Autodesk Inventor part; units mm, degrees
ref_plane "YZ Plane" through (0, 0, 0) normal (1, 0, 0) x (0, 1, 0)
ref_plane "XZ Plane" through (0, 0, 0) normal (0, 1, 0) x (-1, 0, 0)
ref_plane "XY Plane" through (0, 0, 0) normal (0, 0, 1) x (1, 0, 0)
sketch "Esquisse2" plane through (0, 0, 0) normal (1, 0, 0) x (0, 1, 0)
  line L0 (0, 0) -> (0, -2.1683)
  line L1 (0, 0) -> (0, 50)
  line L2 (0, 0) -> (1.5, 0)
  line L3 (1.5, 0) -> (1.5, 5)
  line L4 (1.5, 5) -> (2.5, 5)
  line L5 (2.5, 5) -> (2.5, 10)
  line L6 (2.5, 10) -> (1.5, 10)
  line L7 (1.5, 10) -> (1.5, 50)
  line L8 (0, 50) -> (1.5, 50)
  dimension "d0" = 3
  dimension "d1" = 1
  dimension "d2" = 5
  dimension "d3" = 5
  dimension "d4" = 40
revolve "Révolution1" add sketch "Esquisse2" angle 360 about axis through (0, 0, 0) along (0, 0, -1)
thread "Filetage1"
chamfer "Chanfrein1" distance 0.5 angle 45 1 edges at (0, -1.5, 0)
properties part number "piston_axe"
The model under review builds one solid part; all positions refer to its coordinate system, in mm. A direction names the side the tool comes from. Coordinates: 2 decimals unless noted, no trailing zeros. Write each loop counter-clockwise with the first axis right and the second up, starting at its lowest first coordinate (ties: lowest second). Pieces come first, ordered by that corner, then holes. Notation, with made-up numbers: (75, 78) -> (113, 78) arc R15 ccw to (113, 82) -> close; hole circle Ø7 at (69.25, 66). An arc over 180 degrees is marked (long way). One line per item, written item: value. Start each with the question number.
Q1. To check wall thickness, follow probe 1 along Y at (x, z) = (0.05, 46.5); probe 2 along Z at (x, y) = (-1.5, 1.35); probe 3 along X at (y, z) = (-0.55, 25). State the ranges of each line that lie inside material, in increasing order.
Q2. For faces 3 (the face through (0, 2, 5)), 4 (the face through (0, 0, 50)), 5 (the face through (0, 2, 10)), list the 3-axis set-ups (+Z, -Z, +X, -X, +Y, -Y) from which the entire face can be reached by the end or side of a thin tool; tool diameter is ignored.
Q3. Add section A-A, the plane y = 0. Give the boundary of the cut face in (x, z).
Q4. The part is to be moulded in two halves that separate along Y. For faces 1 (the face through (0, 0, 0)), 2 (the face through (2.44, -0.54, 7.54)), say which applies: +Y half, -Y half, draft (parallel to the pull), parting line (faces both ways), or undercut.
Q5. Add section C-C, the plane z = 27. Give the boundary of the cut face in (x, y).
Q6. Add section D-D, the plane x = -2. Give the boundary of the cut face in (y, z), then the cut area to 3 significant figures.
Q7. Clearance check with flat-ended pins moving along their axes: P1, Ø2, axis at x = 2, z = 16.5, coming from the -Y side; P2, Ø3, axis at y = 0.5, z = 39.5, coming from the -X side; P3, Ø1.5, axis at x = 1, z = 29, coming from the -Y side. State where each tip first meets the part, or that it passes through.
Response:
1. probe 1: -1.5 to 1.5
1. probe 2: 5 to 10
1. probe 3: -1.4 to 1.4
2. face 3: -Z
2. face 4: +Z, +X, -X, +Y, -Y
2. face 5: +Z
3. outline: (-2.5, 5) -> (-1.5, 5) -> (-1.5, 0.5) -> (-1, 0) -> (1, 0) -> (1.5, 0.5) -> (1.5, 5) -> (2.5, 5) -> (2.5, 10) -> (1.5, 10) -> (1.5, 50) -> (-1.5, 50) -> (-1.5, 10) -> (-2.5, 10) -> close
4. face 1: draft
4. face 2: parting line
5. outline: circle Ø3 at (0, 0)
6. outline: (-1.5, 5) -> (1.5, 5) -> (1.5, 10) -> (-1.5, 10) -> close
6. area: 15.0 mm²
7. P1: y = -1.12
7. P2: x = -1.5
7. P3: y = -1.48
